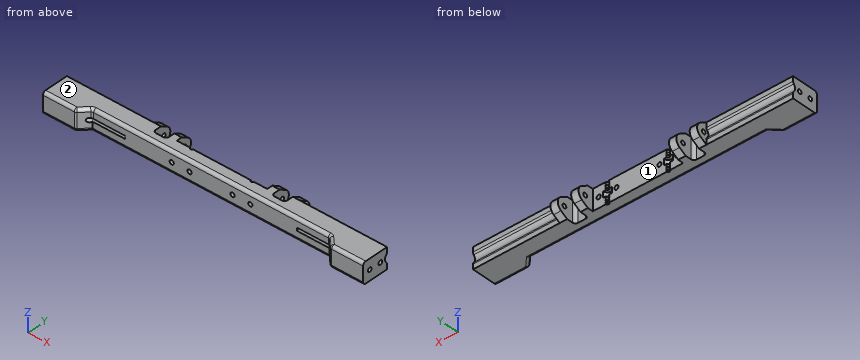
from build123d import *

# Parameters (mm, degrees)
SKETCH1_W           = 17.78
SKETCH1_H           = 22.86
BOSS_EXTRUDE1_DEPTH = 137.16
SKETCH3_R           = 1.778
CUT_EXTRUDE2_DEPTH  = 63.5
SKETCH4_R           = 1.778
BOSS_EXTRUDE2_DEPTH = 6.35
CUT_EXTRUDE3_DEPTH  = 11.43
CUT_EXTRUDE5_DEPTH  = 140.792333123
SKETCH8_R           = 1.778
CUT_EXTRUDE6_DEPTH  = 139.642416385
BOSS_EXTRUDE3_DEPTH = 0.635
LPATTERN1_COUNT     = 10
LPATTERN1_PITCH     = 1.905
SKETCH10_R          = 3.81
CUT_EXTRUDE7_DEPTH  = 2.54
SKETCH11_R          = 4.445
CUT_EXTRUDE8_DEPTH  = 202.250925774
SKETCH12_W          = 203.2
SKETCH12_H          = 7.62
CUT_EXTRUDE9_DEPTH  = 140.792333123
CHAMFER1_SIZE       = 7.62
FILLET1_R           = 2.54


# Read off the part's stored shape, not the designer's step: Mirror2
with BuildPart() as part:
    # Sketch1 → Boss-Extrude1 (new, symmetric)
    with BuildSketch(Plane(origin=(0, 0, 0), x_dir=(0, 0, -1), z_dir=(1, 0, 0))):
        Rectangle(SKETCH1_W, SKETCH1_H)
    extrude(amount=BOSS_EXTRUDE1_DEPTH, both=True)

    # Sketch3 → Cut-Extrude2 (cut)
    with BuildSketch(Plane(origin=(137.16, 0, 0), x_dir=(0, 0, -1), z_dir=(1, 0, 0))):
        with Locations((0, -5.08)):
            Circle(SKETCH3_R)
        with Locations(Location((0, 5.08, 0), (0, 0, 180))):
            Circle(SKETCH3_R)
    extrude(amount=-CUT_EXTRUDE2_DEPTH, mode=Mode.SUBTRACT)

    # Sketch4 → Boss-Extrude2 (add)
    with BuildSketch(Plane(origin=(56.515, 0, 0), x_dir=(0, 0, -1), z_dir=(1, 0, 0))):
        with BuildLine():
            Line((-8.89, 11.43), (-5.461360062, 17.209760218))
            ThreePointArc((-5.461360062, 17.209760218), (0, 20.32), (5.461360062, 17.209760218))
            Line((5.461360062, 17.209760218), (8.89, 11.43))
            Line((8.89, 11.43), (-8.89, 11.43))
        make_face()
        with Locations((0, 13.97)):
            Circle(SKETCH4_R, mode=Mode.SUBTRACT)
    boss_extrude2 = extrude(amount=BOSS_EXTRUDE2_DEPTH)

    # Mirror1: Boss-Extrude2 across plane
    add(boss_extrude2.mirror(Plane.ZY.offset(-50.8)))

    # Sketch5 → Cut-Extrude3 (cut)
    with BuildSketch(Plane(origin=(56.515, 0, 0), x_dir=(0, 0, -1), z_dir=(1, 0, 0))):
        with BuildLine():
            Line((-10.16, 13.97), (-10.16, 3.81))
            Line((-10.16, 3.81), (10.16, 3.81))
            Line((10.16, 3.81), (10.16, 13.97))
            ThreePointArc((10.16, 13.97), (0, 24.13), (-10.16, 13.97))
        make_face()
    extrude(amount=-CUT_EXTRUDE3_DEPTH, mode=Mode.SUBTRACT)

    # Sketch6 → Cut-Extrude5 (cut, through all)
    with BuildSketch(Plane.XY.offset(8.89)):
        with BuildLine():
            ThreePointArc((24.403655463, 6.731), (26.035, 5.334), (27.666344537, 6.731))
            Line((27.666344537, 6.731), (24.403655463, 6.731))
        make_face()
        with BuildLine():
            Line((24.403655463, 6.731), (27.666344537, 6.731))
            ThreePointArc((27.666344537, 6.731), (27.6810788, 6.857620314), (27.686, 6.985))
            ThreePointArc((27.686, 6.985), (25.907620314, 8.6310788), (24.403655463, 6.731))
        make_face()
        with BuildLine():
            Line((27.666344537, 6.731), (38.735, 6.731))
            Line((38.735, 6.731), (38.735, 11.43))
            Line((38.735, 11.43), (0, 11.43))
            Line((0, 11.43), (0, 6.731))
            Line((0, 6.731), (24.403655463, 6.731))
            ThreePointArc((24.403655463, 6.731), (25.907620314, 8.6310788), (27.686, 6.985))
            ThreePointArc((27.686, 6.985), (27.6810788, 6.857620314), (27.666344537, 6.731))
        make_face()
    extrude(amount=-CUT_EXTRUDE5_DEPTH, mode=Mode.SUBTRACT)

    # Sketch8 → Cut-Extrude6 (cut, through all)
    with BuildSketch(Plane(origin=(0, 6.731, 0), x_dir=(1, 0, 0), z_dir=(0, 1, 0))):
        with Locations(Location((18.415, 0, 0), (0, 0, 180))):
            Circle(SKETCH8_R)
        with Locations((33.655, 0)):
            Circle(SKETCH8_R)
    extrude(amount=-CUT_EXTRUDE6_DEPTH, mode=Mode.SUBTRACT)

    # Sketch9 → Boss-Extrude3 (add)
    with BuildSketch(Plane.XY.offset(8.89)):
        with BuildLine():
            Line((24.403655463, 6.731), (24.661284964, 6.731))
            ThreePointArc((24.661284964, 6.731), (26.035, 5.588), (27.408715036, 6.731))
            Line((27.408715036, 6.731), (27.666344537, 6.731))
            ThreePointArc((27.666344537, 6.731), (26.035, 5.334), (24.403655463, 6.731))
        make_face()
    boss_extrude3 = extrude(amount=-BOSS_EXTRUDE3_DEPTH)

    # LPattern1: Boss-Extrude3 ×10
    with Locations(*[(0, 0, -i * LPATTERN1_PITCH) for i in range(1, LPATTERN1_COUNT)]):
        add(boss_extrude3)

    # Sketch10 → Cut-Extrude7 (cut, symmetric)
    with BuildSketch(Plane.XY):
        with Locations((26.035, 6.985)):
            Circle(SKETCH10_R)
    extrude(amount=CUT_EXTRUDE7_DEPTH, both=True, mode=Mode.SUBTRACT)

    # Sketch11 → Cut-Extrude8 (cut, through all)
    with BuildSketch(Plane(origin=(62.865, 0, 0), x_dir=(0, 0, -1), z_dir=(1, 0, 0))):
        with Locations((0, 13.97)):
            Circle(SKETCH11_R)
    extrude(amount=CUT_EXTRUDE8_DEPTH, mode=Mode.SUBTRACT)

    # Mirror2
    split(bisect_by=Plane(origin=(0, 0, 0), x_dir=(0, 0, 1), z_dir=(1, 0, 0)), keep=Keep.TOP)

    # Mirror2 2: part across plane


with BuildPart() as part_1:
    add(part.part)
    add(part.part.mirror(Plane(origin=(0, 0, 0), x_dir=(0, 0, 1), z_dir=(1, 0, 0))))

    # Sketch12 → Cut-Extrude9 (cut, through all)
    with BuildSketch(Plane(origin=(0, 0, -8.89), x_dir=(-1, 0, 0), z_dir=(0, 0, -1))):
        with Locations((0, -7.62)):
            Rectangle(SKETCH12_W, SKETCH12_H)
    extrude(amount=-CUT_EXTRUDE9_DEPTH, mode=Mode.SUBTRACT)

    # Chamfer1
    # the kernel refuses this chamfer: 7.62 mm, written as the material it takes off along each edge
    with BuildSketch(Plane(origin=(-101.6, -11.43, -28.486224368), x_dir=(-0.9996219169112968, -0.02749587661058636, 0), z_dir=(0, 0, 1))) as chamfer1_piece_1:
        Polygon((CHAMFER1_SIZE * 0.999621916911, -CHAMFER1_SIZE * 0.0274958766106), (-CHAMFER1_SIZE * 0.0274958766106, -CHAMFER1_SIZE * 0.999621916911), (0, 0), align=None)
    extrude(amount=56.972448737, mode=Mode.SUBTRACT)
    with BuildSketch(Plane(origin=(101.6, -11.43, -28.486224368), x_dir=(0.9996219169112968, -0.02749587661058636, 0), z_dir=(0, 0, 1))) as chamfer1_piece_2:
        Polygon((CHAMFER1_SIZE * 0.999621916911, CHAMFER1_SIZE * 0.0274958766106), (-CHAMFER1_SIZE * 0.0274958766106, CHAMFER1_SIZE * 0.999621916911), (0, 0), align=None)
    extrude(amount=56.972448737, mode=Mode.SUBTRACT)

    # Fillet1
    fillet1_edges = [part_1.edges().sort_by_distance(p)[0] for p in [
        (100.0125, 11.43, -3.647797281),
        (100.0125, 11.43, 3.647797281),
        (-56.515, 3.81, 0),
        (-45.085, 3.81, 0),
        (-100.0125, 11.43, 3.647797281),
        (-100.0125, 11.43, -3.647797281),
        (101.6, -3.81, 5.067170395),
        (0, -3.81, 8.89),
        (-101.6, -3.81, 5.067170395),
        (0, -3.81, -8.89),
        (123.19, -11.43, -8.89),
        (105.41, -7.62, -8.89),
        (-105.41, -7.62, -8.89),
        (-109.22, -11.43, 0),
        (123.19, -11.43, 8.89),
        (105.41, -7.62, 8.89),
        (-105.41, -7.62, 8.89),
        (109.22, -11.43, 0),
        (56.515, 3.81, 0),
        (45.085, 3.81, 0),
        (-123.19, -11.43, -8.89),
        (-123.19, -11.43, 8.89),
    ]]
    fillet(fillet1_edges, radius=FILLET1_R)


solid = part_1.part
Source: CAD feature listing. Evaluate the final solid. Frame: model axes, mm. Face numbers are marked on the shaded views. Coordinates: 2 decimals unless noted, no trailing zeros. Write each loop counter-clockwise with the first axis right and the second up, starting at its lowest first coordinate (ties: lowest second). Pieces come first, ordered by that corner, then holes. Notation, with made-up numbers: M 56.5,29.25 L 83.5,29.25 A19 ccw 83.5,49.25 Z; hole C -33,48 d1. An arc over 180 degrees is marked long. Use a Markdown table: item, result.
1) First-contact query: pin 1 Ø1.1 at (x, y) = (-26.5, 6.5) entering from +Z; pin 2 Ø1.2 at (x, z) = (94.5, 7.5) entering from +Y; pin 3 Ø4.5 at (x, z) = (33.655, 0) entering from -Y; pin 4 Ø4.5 at (y, z) = (13.97, 0) entering from +X (3 decimals). Flat tips, straight axial feed; report the tip coordinate or a pass-through.
Conclusion:
| item | result |
|---|---|
| pin 1 | passes through |
| pin 2 | stops at y = 11.43 |
| pin 3 | stops at y = -3.81 |
| pin 4 | stops at x = 62.865 |
2) Ray query, L1, parallel to Y at x = 114, z = 0 (3 decimals); L2, parallel to Z at x = -106, y = -5; L3, parallel to Y at x = 90, z = 0 (3 decimals). Return the intervals inside material, ascending.
Conclusion:
| item | result |
|---|---|
| L1 | y = -11.43 to -6.858, -3.302 to 3.302, 6.858 to 9.525 |
| L2 | z = -8.88 to -1.78, 1.78 to 8.88 |
| L3 | y = -3.302 to 3.302, 6.858 to 9.525 |
3) Section A-A, the plane x = -41.5. Output: boundary loops of the cut face in (y, z), then the cut area to 3 significant figures.
Conclusion:
| item | result |
|---|---|
| outline | M -3.81,-6.35 A2.54 ccw -1.27,-8.89 L 11.43,-8.89 L 17.21,-5.46 A6.35 ccw 17.21,5.46 L 11.43,8.89 L -1.27,8.89 A2.54 ccw -3.81,6.35 Z; hole C 13.97,0 d3.56 |
| area | 365 mm^2 |
4) Section B-B, the plane x = -116.5. Output: boundary loops of the cut face in (y, z) (3 decimals), then the cut area to 3 significant figures.
Conclusion:
| item | result |
|---|---|
| outline | M -11.43,-6.35 A2.54 ccw -8.89,-8.89 L 11.43,-8.89 L 11.43,-4.794 A2.54 ccw 10.737,-3.051 A4.445 cw 10.737,3.051 A2.54 ccw 11.43,4.794 L 11.43,8.89 L -8.89,8.89 A2.54 ccw -11.43,6.35 Z; hole C -5.08,0 d3.556; hole C 5.08,0 d3.556 |
| area | 374 mm^2 |
5) Mould query, pull axis X, two halves, no side actions, for the marked faces 1 and 2. Classes: pulls with the +X half, pulls with the -X half, needs draft (parallel to the pull), parting line crosses it, or undercut.
Conclusion:
| item | result |
|---|---|
| face 1 | undercut |
| face 2 | needs draft |
6) Section C-C, the plane x = -78.5. Output: boundary loops of the cut face in (y, z) (3 decimals).
Conclusion:
| item | result |
|---|---|
| outline | M -3.81,-6.35 A2.54 ccw -1.27,-8.89 L 11.43,-8.89 L 11.43,-4.794 A2.54 ccw 10.737,-3.051 A4.445 cw 10.737,3.051 A2.54 ccw 11.43,4.794 L 11.43,8.89 L -1.27,8.89 A2.54 ccw -3.81,6.35 L -3.81,1.244 A1.778 cw -3.81,-1.244 Z; hole C 5.08,0 d3.556 |
